Geometry check sheet. Reference: the model listing, model coordinates, mm. A direction names the side the tool comes from. Round coordinates to 2 decimals unless told otherwise and drop trailing zeros. Loops run counter-clockwise (first coordinate to the right, second up) from the corner with the lowest first, then second, coordinate; pieces in that order, holes last. Notation, with made-up numbers: M -39,-21.75 L -21,-21.75 A8 ccw -21,-11.75 Z; hole C 83,57.5 d6. An arc over 180 degrees is marked long. Use one line per item in the form item = value. Start each with the question number.
1. Go/stop test with flat-tipped pins: pin 1 (6 mm diameter, centred on x = -16.57, y = -23.57, fed in from -Z); pin 2 (3 mm diameter, centred on x = 34, z = -3, fed in from -Y); pin 3 (1.9 mm diameter, centred on x = 4, y = 20, fed in from +Z); pin 4 (3 mm diameter, centred on x = 19, z = -4, fed in from -Y). Record where each tip stops, or that it passes through.
2. Cross-section at B-B (z = -2.75). State how many separate pieces and enclosed holes the cut face has, then the cut area to 3 significant figures.
3. Draft check along Y on faces 1 (the cylindrical face through (-13.523, 16.566, -2.03)), 2 (the flat face through (-22.862, 0, 5)), 3 (the cylindrical face through (-3.47, 11.13, -2.68)), 4 (the flat face through (-18.1, 0, 5)). Enter one of: pulls with the +Y half, pulls with the -Y half, needs draft (parallel to the pull), parting line crosses it, or undercut.
4. Cross-section at A-A (y = 12). Record the boundary of the cut face in (x, z).
5. Cross-section at C-C (x = 30). Record the boundary of the cut face in (y, z), then the cut area to 3 significant figures.
6. Material ranges on line 1 (Z direction, x = -5.5, y = 27); line 2 (Y direction, x = 4.5, z = -2.75); line 3 (X direction, y = 22.5, z = -4), recorded low to high.
7. Set-up check for faces 5 (the flat face through (23.5, 2.3, -2)), 6 (the cylindrical face through (-0.559, -5.796, 5.012)), 7 (the cylindrical face through (6.173, 23.568, -2.03)), 8 (the flat face through (0, -22, 3.04)): record each of +Z, -Z, +X, -X, +Y, -Y from which the full face is reachable in a straight line by a thin tool's end or side.
8. Cross-section at D-D (y = 0). Record the boundary of the cut face in (x, z), then the cut area to 3 significant figures.
```python
from build123d import *

# Parameters (mm, degrees)
SKETCH3_R             = 6.35
SKETCH3_R_2           = 3.175
SKETCH3_R_3           = 2.54
BOSS_EXTRUDE1_DEPTH   = 10
SKETCH2_R             = 2.54
SKETCH2_R_2           = 9.525
SKETCH2_R_3           = 6.35
SKETCH2_R_4           = 3.175
BOSS_EXTRUDE2_DEPTH   = 4
BODY_MOVE_COPY1_ANGLE = 180
SKETCH6_R             = 2.38125
CUT_EXTRUDE1_DEPTH    = 60
BODY_MOVE_COPY2_ANGLE = 90


with BuildPart() as part:
    # Sketch3 → Boss-Extrude1 (new body)
    with BuildSketch(Plane(origin=(0, 0, 0), x_dir=(0, 0, -1), z_dir=(1, 0, 0))):
        with BuildLine():
            Line((19.772410398, 15.481894129), (11.232662335, -18.916334544))
            ThreePointArc((11.232662335, -18.916334544), (0.02933332, -21.999989892), (-11.182178927, -18.946220999))
            Line((-11.182178927, -18.946220999), (-19.828177454, 15.48706861))
            ThreePointArc((-19.828177454, 15.48706861), (-20.537949261, 16.577044264), (-21.767962021, 17))
            Line((-21.767962021, 17), (-32.5, 17))
            Line((-32.5, 17), (-32.5, 26))
            ThreePointArc((-32.5, 26), (-31.328427125, 28.828427125), (-28.5, 30))
            Line((-28.5, 30), (28.5, 30))
            ThreePointArc((28.5, 30), (31.328427125, 28.828427125), (32.5, 26))
            Line((32.5, 26), (32.5, 17))
            Line((32.5, 17), (21.713486916, 17))
            ThreePointArc((21.713486916, 17), (20.481372526, 16.575402846), (19.772410398, 15.481894129))
        make_face()
        Circle(SKETCH3_R, mode=Mode.SUBTRACT)
        with Locations((0, 17.272)):
            Circle(SKETCH3_R, mode=Mode.SUBTRACT)
        with Locations((0, -14.415625)):
            Circle(SKETCH3_R_2, mode=Mode.SUBTRACT)
        with Locations((-23.5712, 23.5712)):
            Circle(SKETCH3_R_3, mode=Mode.SUBTRACT)
        with Locations((23.5712, 23.5712)):
            Circle(SKETCH3_R_3, mode=Mode.SUBTRACT)
    extrude(amount=BOSS_EXTRUDE1_DEPTH)

    # Sketch2 → Boss-Extrude2 (add)
    with BuildSketch(Plane(origin=(10, 0, 0), x_dir=(0, 0, -1), z_dir=(1, 0, 0))):
        with BuildLine():
            Line((-28.5, 30), (28.5, 30))
            ThreePointArc((28.5, 30), (31.328427125, 28.828427125), (32.5, 26))
            Line((32.5, 26), (32.5, -26))
            ThreePointArc((32.5, -26), (31.328427125, -28.828427125), (28.5, -30))
            Line((28.5, -30), (-28.5, -30))
            ThreePointArc((-28.5, -30), (-31.328427125, -28.828427125), (-32.5, -26))
            Line((-32.5, -26), (-32.5, 26))
            ThreePointArc((-32.5, 26), (-31.328427125, 28.828427125), (-28.5, 30))
        make_face()
        with Locations((23.5712, 23.5712)):
            Circle(SKETCH2_R, mode=Mode.SUBTRACT)
        with Locations((-23.5712, 23.5712)):
            Circle(SKETCH2_R, mode=Mode.SUBTRACT)
        with Locations((-23.5712, -23.5712)):
            Circle(SKETCH2_R, mode=Mode.SUBTRACT)
        with Locations((23.5712, -23.5712)):
            Circle(SKETCH2_R, mode=Mode.SUBTRACT)
        Circle(SKETCH2_R_2, mode=Mode.SUBTRACT)
        with Locations(Location((0, 17.3355, 0), (0, 0, 180.286480091))):
            Circle(SKETCH2_R_3, mode=Mode.SUBTRACT)
        with Locations((0, -14.415625)):
            Circle(SKETCH2_R_4, mode=Mode.SUBTRACT)
        with BuildLine():
            Line((-29.8625, -2), (-29.8625, 2))
            ThreePointArc((-29.8625, 2), (-27.48125, 4.38125), (-25.1, 2))
            Line((-25.1, 2), (-25.1, -2))
            ThreePointArc((-25.1, -2), (-27.48125, -4.38125), (-29.8625, -2))
        make_face(mode=Mode.SUBTRACT)
        with BuildLine():
            Line((25.1, -2), (25.1, 2))
            ThreePointArc((25.1, 2), (27.48125, 4.38125), (29.8625, 2))
            Line((29.8625, 2), (29.8625, -2))
            ThreePointArc((29.8625, -2), (27.48125, -4.38125), (25.1, -2))
        make_face(mode=Mode.SUBTRACT)
    extrude(amount=BOSS_EXTRUDE2_DEPTH)


with BuildPart() as part_1:
    # Body-Move/Copy1: moved
    add(part.part.rotate(Axis((7, 0, 0.02), (0, 1, 0)), BODY_MOVE_COPY1_ANGLE))

    # Sketch6 → Cut-Extrude1 (cut)
    with BuildSketch(Plane(origin=(0, 30, 0), x_dir=(-1, 0, 0), z_dir=(0, 1, 0))):
        with Locations(Location((-8.999786825, -12.69999899, 0), (0, 0, 90))):
            Circle(SKETCH6_R)
        with Locations(Location((-9.00991527, 12.69999899, 0), (0, 0, 90))):
            Circle(SKETCH6_R)
    extrude(amount=-CUT_EXTRUDE1_DEPTH, mode=Mode.SUBTRACT)


with BuildPart() as part_2:
    # Body-Move/Copy2: moved
    add(part_1.part.rotate(Axis((7.0000125, 0, 0.04), (0, 1, 0)), BODY_MOVE_COPY2_ANGLE))


solid = part_2.part
```
Reported:
q1.pin_1 = 3.04
q1.pin_2 = 17
q1.pin_3 = through
q1.pin_4 = -19.33
q2.separate_pieces = 3
q2.enclosed_holes = 5
q2.area = 1,300 mm²
q3.face_1 = pulls with the -Y half
q3.face_2 = undercut
q3.face_3 = needs draft
q3.face_4 = undercut
q4.outline = M -25.5,3.04 L -11.95,3.04 L -11.95,-6.96 L 3.46,-6.96 L 3.46,3.04 L 3.56,3.04 L 3.56,7.04 L -25.5,7.04 Z; M 10.44,3.04 L 10.54,3.04 L 10.54,-6.96 L 25.91,-6.96 L 25.91,3.04 L 39.5,3.04 L 39.5,7.04 L 10.44,7.04 Z; hole C -5.74,-1.96 d4.76; hole C 19.66,-1.97 d4.76
q5.outline = M -30,3.04 L -26.05,3.04 L -26.05,7.04 L -30,7.04 Z; M -21.1,3.04 L 17,3.04 L 17,-6.96 L 21.1,-6.96 L 21.1,7.04 L -21.1,7.04 Z; M 26.05,-6.96 L 30,-6.96 L 30,7.04 L 26.05,7.04 Z
q5.area = 281 mm²
q6.line_1 = -6.96 to -4.33, 0.41 to 7.04
q6.line_2 = -21.86 to -16.37, -12.46 to -5.84, 5.84 to 11.43, 23.11 to 30
q6.line_3 = -25.5 to -18.87, -14.27 to -6.97, -4.51 to 3.4, 10.6 to 18.42, 20.9 to 28.27, 32.87 to 39.5
q7.face_5 = -Z, +X, -Y
q7.face_6 = +Z
q7.face_7 = -Z
q7.face_8 = -Z, -Y
q8.outline = M -25.5,3.04 L -22.86,3.04 L -22.86,7.04 L -25.5,7.04 Z; M -18.1,3.04 L -8.94,3.04 L -8.94,-6.96 L 0.65,-6.96 L 0.65,3.04 L -2.52,3.04 L -2.52,7.04 L -18.1,7.04 Z; M 13.35,-6.96 L 22.93,-6.96 L 22.93,3.04 L 32.1,3.04 L 32.1,7.04 L 16.53,7.04 L 16.53,3.04 L 13.35,3.04 Z; M 36.86,3.04 L 39.5,3.04 L 39.5,7.04 L 36.86,7.04 Z; hole C -5.74,-1.96 d4.76; hole C 19.66,-1.97 d4.76
q8.area = 302 mm²
